from build123d import *

# Parameters (mm, degrees)
SKETCH_1_R          = 24
EXTRUDE_1_DEPTH     = 10
SKETCH_2_R          = 14
EXTRUDE_2_DEPTH     = 10
SKETCH_3_R          = 13.9
EXTRUDE_3_DEPTH     = 22
CUT_EXTRUDE_START   = -22
CUT_EXTRUDE_1_DEPTH = 22
SKETCH_5_R          = 2.75
CUT_EXTRUDE_2_DEPTH = 22
SKETCH_6_R          = 8
CUT_EXTRUDE_3_DEPTH = 53.345009313


with BuildPart() as part:
    # 스케치1 → 보스-돌출1 (new body)
    with BuildSketch(Plane.XY):
        Circle(SKETCH_1_R)
    extrude(amount=EXTRUDE_1_DEPTH)

    # 스케치2 → 보스-돌출2 (add)
    with BuildSketch(Plane(origin=(0, 0, 0), x_dir=(-1, 0, 0), z_dir=(0, 0, -1))):
        Circle(SKETCH_2_R)
    extrude(amount=EXTRUDE_2_DEPTH)

    # 스케치3 → 보스-돌출3 (add)
    with BuildSketch(Plane(origin=(0, 0, -10), x_dir=(-1, 0, 0), z_dir=(0, 0, -1))):
        Circle(SKETCH_3_R)
    extrude(amount=EXTRUDE_3_DEPTH)

    # 스케치4 → 컷-돌출1 (cut)
    with BuildSketch(Plane.XY.offset(10).offset(CUT_EXTRUDE_START)):
        with BuildLine():
            ThreePointArc((24, 0), (22.978250586, 6.92820323), (20, 13.266499161))
            Line((20, 13.266499161), (20, -13.266499161))
            ThreePointArc((20, -13.266499161), (22.978250586, -6.92820323), (24, 0))
        make_face()
        with BuildLine():
            Line((-20, -13.266499161), (-20, 13.266499161))
            ThreePointArc((-20, 13.266499161), (-24, 0), (-20, -13.266499161))
        make_face()
    extrude(amount=CUT_EXTRUDE_1_DEPTH, mode=Mode.SUBTRACT)

    # 스케치5 → 컷-돌출2 (cut)
    with BuildSketch(Plane.XY.offset(10)):
        with Locations((0, 19)):
            Circle(SKETCH_5_R)
        with Locations((-13.435028843, 13.435028843)):
            Circle(SKETCH_5_R)
        with Locations((13.435028843, 13.435028843)):
            Circle(SKETCH_5_R)
        with Locations((13.435028843, -13.435028843)):
            Circle(SKETCH_5_R)
        with Locations((0, -19)):
            Circle(SKETCH_5_R)
        with Locations((-13.435028843, -13.435028843)):
            Circle(SKETCH_5_R)
    extrude(amount=-CUT_EXTRUDE_2_DEPTH, mode=Mode.SUBTRACT)

    # 스케치6 → 컷-돌출3 (cut, through all)
    with BuildSketch(Plane.XY.offset(10)):
        Circle(SKETCH_6_R)
    extrude(amount=-CUT_EXTRUDE_3_DEPTH, mode=Mode.SUBTRACT)


solid = part.part
Verification items for the finished model (mm, model axes). A direction names the side the tool comes from. Coordinates: 2 decimals unless noted, no trailing zeros. Loops run counter-clockwise (first coordinate to the right, second up) from the corner with the lowest first, then second, coordinate; pieces in that order, holes last. Notation, with made-up numbers: (-37, -3.75) -> (-12, -3.75) arc R24 ccw to (-12, 31.25) -> close; hole circle Ø8 at (80.5, 51). An arc over 180 degrees is marked (long way). Answer as a JSON object with one key per item and string values. Group by question number.
Item 1: Sectioned sample at D-D on z = 1.5. Record the boundary of the cut face in (x, y), plus the area to 3 significant figures.
Item 2: Sectioned sample at C-C on y = -15.5. Record the boundary of the cut face in (x, z).
Item 3: Sectioned sample at A-A on y = 19. Record the boundary of the cut face in (x, z).
Item 4: Tool access check on faces 4 (the cylindrical face through (-15.462, 15.294, 5.07)), 5 (the cylindrical face through (-12.932, -5.362, -4.93)). Record the directions out of +Z, -Z, +X, -X, +Y, -Y that give a thin tool (end or side, any length) a straight path to the whole face; none if there is none.
Item 5: Sectioned sample at B-B on x = 4. Record the boundary of the cut face in (y, z), plus the area to 3 significant figures.
Item 6: Depth check by flat-ended pin: pin 1 (5 mm diameter, centred on x = -8.5, z = -3, fed in from -Y); pin 2 (4 mm diameter, centred on x = -5, z = -17, fed in from -Y); pin 3 (18.5 mm diameter, centred on x = 0, y = 0, fed in from +Z); pin 4 (6.5 mm diameter, centred on x = 13.44, y = -13.44, fed in from -Z). Enter the tip coordinate at first touch or a pass-through.
Item 7: Scan lines: probe 1 along Y at (x, z) = (1.5, 3); probe 2 along X at (y, z) = (-12, 1); probe 3 along Z at (x, y) = (-16, -1). Record each from-to range of solid material in increasing order.
Item 8: Mould release check, pull along Y, two halves, no side actions. Record for faces 1 (the cylindrical face through (0, 24, 5)), 2 (the cylindrical face through (10.688, -13.314, 5.07)), 3 (the flat face through (-9, 11, 0)): +Y half, -Y half, draft (parallel to the pull), parting line (faces both ways), or undercut.
Evaluation:
{
 "1": {"outline": "(-20, -13.27) arc R24 ccw to (20, -13.27) -> (20, 13.27) arc R24 ccw to (-20, 13.27) -> close; hole circle Ø5.5 at (-13.44, -13.44); hole circle Ø5.5 at (-13.44, 13.44); hole circle Ø16 at (0, 0); hole circle Ø5.5 at (0, -19); hole circle Ø5.5 at (0, 19); hole circle Ø5.5 at (13.44, -13.44); hole circle Ø5.5 at (13.44, 13.44)", "area": "1,320 mm²"},
 "2": {"outline": "(-18.32, 0) -> (-15.25, 0) -> (-15.25, 10) -> (-18.32, 10) -> close; (-11.62, 0) -> (11.62, 0) -> (11.62, 10) -> (-11.62, 10) -> close; (15.25, 0) -> (18.32, 0) -> (18.32, 10) -> (15.25, 10) -> close"},
 "3": {"outline": "(-14.66, 0) -> (-2.75, 0) -> (-2.75, 10) -> (-14.66, 10) -> close; (2.75, 0) -> (14.66, 0) -> (14.66, 10) -> (2.75, 10) -> close"},
 "4": {"face 4": "+Z, -Z", "face 5": "-Z"},
 "5": {"outline": "(-23.66, 0) -> (-13.42, 0) -> (-13.42, -10) -> (-13.31, -10) -> (-13.31, -32) -> (-6.93, -32) -> (-6.93, 10) -> (-23.66, 10) -> close; (6.93, -32) -> (13.31, -32) -> (13.31, -10) -> (13.42, -10) -> (13.42, 0) -> (23.66, 0) -> (23.66, 10) -> (6.93, 10) -> close", "area": "745 mm²"},
 "6": {"pin 1": "stops at y = -12.65", "pin 2": "stops at y = -13.57", "pin 3": "stops at z = 10", "pin 4": "stops at z = 0"},
 "7": {"probe 1": "y = -23.95 to -21.3, -16.7 to -7.86, 7.86 to 16.7, 21.3 to 23.95", "probe 2": "x = -20 to -15.78, -11.09 to 11.09, 15.78 to 20", "probe 3": "z = 0 to 10"},
 "8": {"face 1": "+Y half", "face 2": "undercut", "face 3": "draft"}
}
